Answer from the drawing. Dimensions are ordinates in mm from the lowest x, y and z of the part. A direction names the side the tool comes from. Coordinates: 2 decimals unless noted, no trailing zeros. Write each loop counter-clockwise with the first axis right and the second up, starting at its lowest first coordinate (ties: lowest second). Pieces come first, ordered by that corner, then holes. Notation, with made-up numbers: (-4.75, 86) -> (20.25, 86) arc R18 ccw to (20.25, 103) -> close; hole circle Ø10 at (47.5, 41.5). An arc over 180 degrees is marked (long way). Return JSON: item names as keys, results as strings.
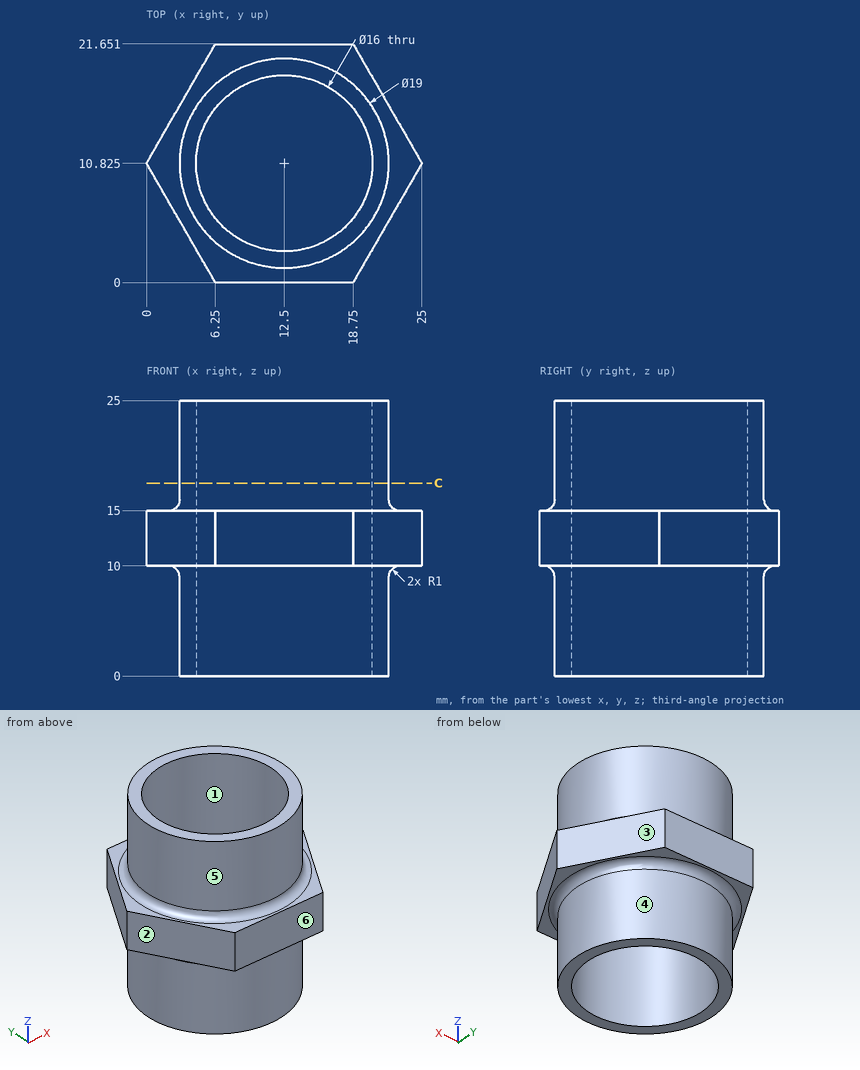
1. For a pull along Y with two mould halves and no side action, classify the marked faces 1, 2, 3 and 4 as +Y half, -Y half, draft (parallel to the pull), parting line (faces both ways), or undercut.
Taken from the geometry:
{"face 1": "undercut", "face 2": "-Y half", "face 3": "+Y half", "face 4": "parting line"}
2. Flat-ended cylindrical pins translate along their axes: pin 1 Ø11 at (x, y) = (13, 10) entering from -Z; pin 2 Ø6 at (x, y) = (20, 9.5) entering from -Z; pin 3 Ø1.5 at (x, z) = (19.5, 7.5) entering from +Y. Find the tip coordinate at first contact, or state that the pin passes through.
Taken from the geometry:
{"pin 1": "passes through", "pin 2": "stops at z = 0", "pin 3": "stops at y = 17.98"}
3. Consider L1, parallel to Y at x = 12.25, z = 22.25; L2, parallel to X at y = 10.5, z = 4.25 (1 decimal); L3, parallel to X at y = 11, z = 15.5. Determine where each line is inside the solid, lowest interval first.
Taken from the geometry:
{"L1": "y = 1.33 to 2.83, 18.82 to 20.32", "L2": "x = 3 to 4.5, 20.5 to 22", "L3": "x = 2.87 to 4.5, 20.5 to 22.13"}
4. A tool of negligible diameter and unlimited length cuts with its end or side. For the marked faces 5 and 6, from which of +Z, -Z, +X, -X, +Y, -Y can it reach the whole face along a straight path? Write none if from no direction.
Taken from the geometry:
{"face 5": "+Z", "face 6": "+Z, -Z, +X, -X, -Y"}
5. The part is cut by section C-C (z = 17.5). Determine the outline of the cut face in (x, y) (1 decimal).
Taken from the geometry:
{"outline": "circle Ø19 at (12.5, 10.8); hole circle Ø16 at (12.5, 10.8)"}
